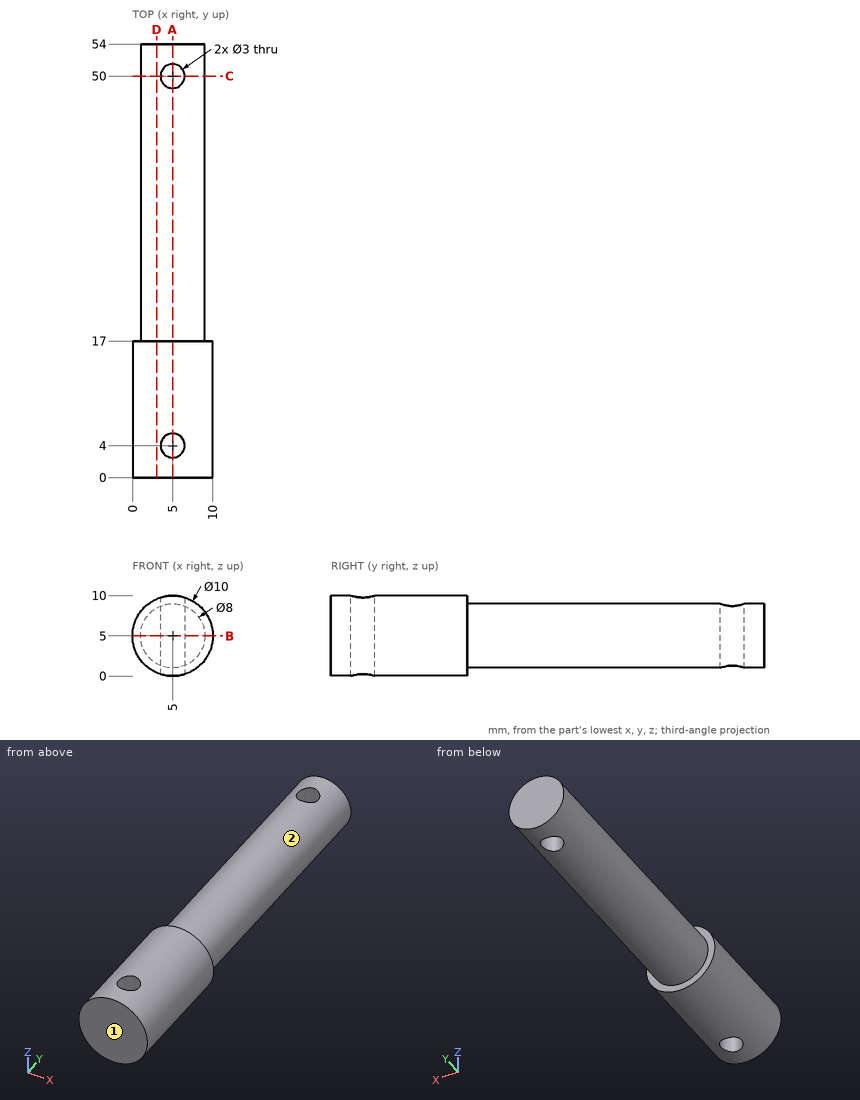
Check sheet for the drawn part. Datum: minimum x, y, z corner. Units: mm. A direction names the side the tool comes from. Round coordinates to 2 decimals unless told otherwise and drop trailing zeros. Loops run counter-clockwise (first coordinate to the right, second up) from the corner with the lowest first, then second, coordinate; pieces in that order, holes last. Notation, with made-up numbers: (-34, 1) - (-6, 1) arc R10 cw to (-6, 9) - close; hole circle Ø4 at (-31.75, -13.5). An arc over 180 degrees is marked (long way). Write item = value, one per line. Start each with the question number.
1. Section check B-B on z = 5. Enter the section's corners in (x, y).
2. Section check A-A on x = 5. Enter the section's corners in (y, z), then the cut area to 3 significant figures.
3. Set-up check for the marked faces 1 and 2: record each of +Z, -Z, +X, -X, +Y, -Y from which the full face is reachable in a straight line by a thin tool's end or side.
4. Section check D-D on x = 3. Enter the section's corners in (y, z).
5. Depth check by flat-ended pin: pin 1 (1 mm diameter, centred on y = 31, z = 9, fed in from +X); pin 2 (5 mm diameter, centred on x = 2.5, y = 36.5, fed in from +Z); pin 3 (2.5 mm diameter, centred on x = 5, y = 4, fed in from +Z); pin 4 (5 mm diameter, centred on y = 46.5, z = 3, fed in from -X). Enter the tip coordinate at first touch or a pass-through.
6. Thickness scan on line 1 (Y direction, x = 5, z = 6); line 2 (Y direction, x = 6.25, z = 2.25); line 3 (Z direction, x = 5.25, y = 44.5). Record the ranges inside material, lowest first.
7. Section check C-C on y = 50. Enter the section's corners in (x, z), then the cut area to 3 significant figures.
Working result:
q1.outline = (0, 0) - (10, 0) - (10, 17) - (9, 17) - (9, 54) - (1, 54) - (1, 17) - (0, 17) - close; hole circle Ø3 at (5, 4); hole circle Ø3 at (5, 50)
q2.outline = (0, 0) - (2.5, 0) - (2.5, 10) - (0, 10) - close; (5.5, 0) - (17, 0) - (17, 1) - (48.5, 1) - (48.5, 9) - (17, 9) - (17, 10) - (5.5, 10) - close; (51.5, 1) - (54, 1) - (54, 9) - (51.5, 9) - close
q2.area = 412 mm^2
q3.face_1 = +Z, -Z, +X, -X, -Y
q3.face_2 = +Y
q4.outline = (0, 0.42) - (17, 0.42) - (17, 1.54) - (54, 1.54) - (54, 8.46) - (17, 8.46) - (17, 9.58) - (0, 9.58) - close
q5.pin_1 = 6.94
q5.pin_2 = 9
q5.pin_3 = through
q5.pin_4 = 1
q6.line_1 = 0 to 2.5, 5.5 to 48.5, 51.5 to 54
q6.line_2 = 0 to 3.17, 4.83 to 49.17, 50.83 to 54
q6.line_3 = 1.01 to 8.99
q7.outline = (3.5, 1.29) - (3.5, 8.71) arc R4 ccw to start; (6.5, 1.29) arc R4 ccw to (6.5, 8.71) - close
q7.area = 26.8 mm^2
